The listing builds one solid part. Answer for the finished solid, in the listing's coordinates (mm). A direction names the side the tool comes from. Round coordinates to 2 decimals unless told otherwise and drop trailing zeros. Write each loop counter-clockwise with the first axis right and the second up, starting at its lowest first coordinate (ties: lowest second). Pieces come first, ordered by that corner, then holes. Notation, with made-up numbers: (-28.75, 61.25) - (-12.75, 61.25) arc R32 ccw to (-12.75, 90.25) - close; hole circle Ø5 at (-32, -25). An arc over 180 degrees is marked (long way). Use a Markdown table: item, result. Add a question column.
1) Each of these flat-tipped pins is pushed along its axis until it touches: P1, Ø1.5, axis at x = -7.5, y = 14, coming from the -Z side; P2, Ø10, axis at x = 37, y = 40.5, coming from the -Z side; P3, Ø1.7, axis at x = 39, z = 28.5, coming from the +Y side; P4, Ø1.8, axis at y = 40.5, z = 24.5, coming from the +X side. Where does it stop, or does it pass through?
2) A cutting plane is placed at D-D (y = 29). Give the vertices of the cut face in (x, z), then the cut area to 3 significant figures.
3) Determine the mould class of faces 1 (the cylindrical face through (-50.07, 2.03, 35.5)), 2 (the cylindrical face through (49.464, 2.028, 0.325)), 3 (the flat face through (-42.5, 33, 0)) for opening direction Z: +Z half, -Z half, draft (parallel to the pull), parting line (faces both ways), or undercut.
4) A cutting plane is placed at C-C (x = -18.5). Give the vertices of the cut face in (y, z).
5) A cutting plane is placed at A-A (x = 0). Give the vertices of the cut face in (y, z).
6) Find the intervals of material crossed by probe 1 along X at (y, z) = (2.2, 0); probe 2 along X at (y, z) = (32.5, 28.5); probe 3 along Z at (x, y) = (5, 40.5), in increasing order. Write a range as from..to.
7) A cutting plane is placed at B-B (z = -5.5). Give the vertices of the cut face in (x, y), then the cut area to 3 significant figures.
8) A tool of negligible diameter and unlimited length cuts with its end or side. For faces 4 (the flat face through (2, 33, 28)), 5 (the flat face through (9, 55, 26)), 6 (the flat face through (-1, 2, 37)), 7 (the flat face through (-51.5, 2, 0)), 8 (the flat face through (38.5, 3, 0)), from which of +Z, -Z, +X, -X, +Y, -Y can it reach the whole face along a straight path? Write none if from no direction.
```python
from build123d import *

# Parameters (mm, degrees)
SKETCH_1_W               = 103
SKETCH_1_H               = 74
EXTRUDE_1_DEPTH          = 4
SKETCH_2_W               = 85
SKETCH_2_H               = 56
EXTRUDE_2_DEPTH          = 56
SKETCH_3_W               = 81
SKETCH_3_H               = 48
CUT_EXTRUDE_1_DEPTH      = 56
SKETCH_7_R               = 4.5
EXTRUDE_3_DEPTH          = 56
SKETCH_8_R               = 1.4
CUT_EXTRUDE_4_DEPTH      = 88.299770905
SKETCH_4_R               = 1.5
CUT_EXTRUDE_2_DEPTH      = 85.600531913
SKETCH_5_W               = 77
SKETCH_5_H               = 48
CUT_EXTRUDE_3_DEPTH      = 26
FILLET_8_R               = 2
FILLET_7_R               = 1
CUT_EXTRUDE_5_DEPTH      = 88.299770973
CUT_EXTRUDE_5_DEPTH_BACK = 88.299770973
SKETCH_9_W               = 50
SKETCH_9_H               = 5
FILLET_9_R               = 5


with BuildPart() as part:
    # 草图1 → 凸台-拉伸1 (new body)
    with BuildSketch(Plane(origin=(0, 0, 0), x_dir=(1, 0, 0), z_dir=(0, 1, 0))):
        Rectangle(SKETCH_1_W, SKETCH_1_H)
    extrude(amount=EXTRUDE_1_DEPTH)

    # 草图2 → 凸台-拉伸2 (add)
    with BuildSketch(Plane(origin=(0, 4, 0), x_dir=(1, 0, 0), z_dir=(0, 1, 0))):
        Rectangle(SKETCH_2_W, SKETCH_2_H)
    extrude(amount=EXTRUDE_2_DEPTH)

    # 草图3 → 切除-拉伸1 (cut)
    with BuildSketch(Plane(origin=(0, 60, 0), x_dir=(1, 0, 0), z_dir=(0, 1, 0))):
        with Locations((2, 0)):
            Rectangle(SKETCH_3_W, SKETCH_3_H)
    extrude(amount=-CUT_EXTRUDE_1_DEPTH, mode=Mode.SUBTRACT)

    # 草图7 → 凸台-拉伸3 (add)
    with BuildSketch(Plane(origin=(0, 4, 0), x_dir=(1, 0, 0), z_dir=(0, 1, 0))):
        with Locations((-35, 28.5)):
            Circle(SKETCH_7_R)
        with Locations((39, 28.5)):
            Circle(SKETCH_7_R)
        with Locations((39, -28.5)):
            Circle(SKETCH_7_R)
        with Locations((-35, -28.5)):
            Circle(SKETCH_7_R)
    extrude(amount=EXTRUDE_3_DEPTH)

    # 草图8 → 切除-拉伸4 (cut, through all)
    with BuildSketch(Plane(origin=(0, 60, 0), x_dir=(1, 0, 0), z_dir=(0, 1, 0))):
        with Locations(Location((-35, 28.5, 0), (0, 0, 270))):
            Circle(SKETCH_8_R)
        with Locations(Location((39, 28.5, 0), (0, 0, 270))):
            Circle(SKETCH_8_R)
        with Locations(Location((-35, -28.5, 0), (0, 0, 270))):
            Circle(SKETCH_8_R)
        with Locations(Location((39, -28.5, 0), (0, 0, 270))):
            Circle(SKETCH_8_R)
    extrude(amount=-CUT_EXTRUDE_4_DEPTH, mode=Mode.SUBTRACT)

    # 草图4 → 切除-拉伸2 (cut, through all)
    with BuildSketch(Plane(origin=(0, 4, 0), x_dir=(1, 0, 0), z_dir=(0, 1, 0))):
        with Locations(Location((-48, 0, 0), (0, 0, 270))):
            Circle(SKETCH_4_R)
        with Locations(Location((48, 0, 0), (0, 0, 90))):
            Circle(SKETCH_4_R)
        with Locations(Location((0, 34, 0), (0, 0, 270))):
            Circle(SKETCH_4_R)
        with Locations(Location((0, -34, 0), (0, 0, 90))):
            Circle(SKETCH_4_R)
    extrude(amount=-CUT_EXTRUDE_2_DEPTH, mode=Mode.SUBTRACT)

    # 草图5 → 切除-拉伸3 (cut)
    with BuildSketch(Plane(origin=(0, 4, 0), x_dir=(1, 0, 0), z_dir=(0, 1, 0))):
        Rectangle(SKETCH_5_W, SKETCH_5_H)
    extrude(amount=-CUT_EXTRUDE_3_DEPTH, mode=Mode.SUBTRACT)

    # 圆角8
    fillet_8_edges = [part.edges().sort_by_distance(p)[0] for p in [
        (40.261608219, 4, -32.819530611),
        (2, 4, -28),
        (-35, 4, -33),
        (-40.986067977, 4, -28),
        (-42.5, 4, 0),
        (-35, 4, 33),
        (40.261608219, 4, 32.819530611),
        (2, 4, 28),
    ]]
    fillet(fillet_8_edges, radius=FILLET_8_R)

    # 圆角7
    fillet_7_edges = [part.edges().sort_by_distance(p)[0] for p in [
        (0, 0, -24),
        (-38.5, 0, 0),
        (38.5, 0, 0),
        (0, 0, 24),
        (2, 60, -24),
        (-38.5, 60, 0),
        (2, 60, 24),
    ]]
    fillet(fillet_7_edges, radius=FILLET_7_R)

    # 草图9 → 切除-拉伸5 (cut, two sides: drawn at the far end of the back side and taken through both)
    with BuildSketch(Plane.XY.offset(-CUT_EXTRUDE_5_DEPTH_BACK)):
        with Locations((9.5, 57.5)):
            Rectangle(SKETCH_9_W, SKETCH_9_H)
    extrude(amount=CUT_EXTRUDE_5_DEPTH + CUT_EXTRUDE_5_DEPTH_BACK, mode=Mode.SUBTRACT)

    # 圆角9
    fillet_9_edges = [part.edges().sort_by_distance(p)[0] for p in [
        (51.5, 2, 37),
        (-51.5, 2, 37),
        (-51.5, 2, -37),
        (51.5, 2, -37),
    ]]
    fillet(fillet_9_edges, radius=FILLET_9_R)


solid = part.part
```
Entries:
| question | item | result |
|---|---|---|
| 1 | P1 | stops at z = -28 |
| 1 | P2 | stops at z = -33 |
| 1 | P3 | passes through |
| 1 | P4 | stops at x = 42.5 |
| 2 | outline | (-42.5, -28) - (-39.47, -28) arc R4.5 ccw (long way) to (-30.53, -28) - (34.53, -28) arc R4.5 ccw (long way) to (42.5, -25.67) - (42.5, -24) - (-38.5, -24) - (-38.5, 24) - (42.5, 24) - (42.5, 25.67) arc R4.5 ccw (long way) to (34.53, 28) - (-30.53, 28) arc R4.5 ccw (long way) to (-39.47, 28) - (-42.5, 28) - close; hole circle Ø2.8 at (-35, -28.5); hole circle Ø2.8 at (-35, 28.5); hole circle Ø2.8 at (39, -28.5); hole circle Ø2.8 at (39, 28.5) |
| 2 | area | 995 mm² |
| 3 | face 1 | +Z half |
| 3 | face 2 | undercut |
| 3 | face 3 | draft |
| 4 | outline | (0, -37) - (4, -37) - (4, -30) arc R2 cw to (6, -28) - (60, -28) - (60, -25) arc R1 ccw to (59, -24) - (1, -24) arc R1 ccw to (0, -25) - close; (0, 25) arc R1 ccw to (1, 24) - (59, 24) arc R1 ccw to (60, 25) - (60, 28) - (6, 28) arc R2 cw to (4, 30) - (4, 37) - (0, 37) - close |
| 5 | outline | (0, -37) - (4, -37) - (4, -35.5) - (0, -35.5) - close; (0, -32.5) - (4, -32.5) - (4, -30) arc R2 cw to (6, -28) - (55, -28) - (55, -24) - (1, -24) arc R1 ccw to (0, -25) - close; (0, 25) arc R1 ccw to (1, 24) - (55, 24) - (55, 28) - (6, 28) arc R2 cw to (4, 30) - (4, 32.5) - (0, 32.5) - close; (0, 35.5) - (4, 35.5) - (4, 37) - (0, 37) - close |
| 6 | probe 1 | x = -51.5..-49.5, -46.5..-38.5, 38.5..46.5, 49.5..51.5 |
| 6 | probe 2 | x = -39.5..-36.4, -33.6..-30.5, 34.5..37.6, 40.4..43.5 |
| 6 | probe 3 | z = -28..-24, 24..28 |
| 7 | outline | (-51.5, 0) - (-39.5, 0) arc R1 ccw to (-38.5, 1) - (-38.5, 59) arc R1 ccw to (-39.5, 60) - (-42.5, 60) - (-42.5, 6) arc R2 cw to (-44.5, 4) - (-51.5, 4) - close; (38.5, 1) arc R1 ccw to (39.5, 0) - (51.5, 0) - (51.5, 4) - (38.5, 4) - close |
| 7 | area | 328 mm² |
| 8 | face 4 | +Z, +Y |
| 8 | face 5 | +Z, -Z, +Y |
| 8 | face 6 | +Z, +X, -X, +Y, -Y |
| 8 | face 7 | +Z, -Z, -X, +Y, -Y |
| 8 | face 8 | +Y, -Y |
